from build123d import *

# Parameters (mm, degrees)
SKETCH_1_R          = 13.05
EXTRUDE_1_DEPTH     = 65.9
SKETCH_2_R          = 10.978194701
CUT_EXTRUDE_1_DEPTH = 0.5
SKETCH_3_R          = 5.021706909
EXTRUDE_2_DEPTH     = 0.5
CUT_EXTRUDE_START   = -0.2
SKETCH_4_R          = 8.048308781
SKETCH_4_R_2        = 5.021706909
CUT_EXTRUDE_2_DEPTH = 0.2


with BuildPart() as part:
    # 草图1 → 凸台-拉伸1 (new body)
    with BuildSketch(Plane(origin=(0, 0, 0), x_dir=(1, 0, 0), z_dir=(0, 1, 0))):
        with Locations(Location((0, 0, 0), (0, 0, 270))):
            Circle(SKETCH_1_R)
    extrude(amount=EXTRUDE_1_DEPTH)

    # 草图2 → 切除-拉伸1 (cut)
    with BuildSketch(Plane.XZ):
        with Locations(Location((0, 0, 0), (0, 0, 270))):
            Circle(SKETCH_2_R)
    extrude(amount=-CUT_EXTRUDE_1_DEPTH, mode=Mode.SUBTRACT)

    # 草图3 → 凸台-拉伸2 (add)
    with BuildSketch(Plane(origin=(0, 65.9, 0), x_dir=(1, 0, 0), z_dir=(0, 1, 0))):
        with Locations(Location((0, 0, 0), (0, 0, 270))):
            Circle(SKETCH_3_R)
    extrude(amount=EXTRUDE_2_DEPTH)

    # 草图4 → 切除-拉伸2 (cut)
    with BuildSketch(Plane(origin=(0, 65.9, 0), x_dir=(1, 0, 0), z_dir=(0, 1, 0)).offset(CUT_EXTRUDE_START)):
        with Locations(Location((0, 0, 0), (0, 0, 270))):
            Circle(SKETCH_4_R)
        with Locations(Location((0, 0, 0), (0, 0, 270))):
            Circle(SKETCH_4_R_2, mode=Mode.SUBTRACT)
    extrude(amount=CUT_EXTRUDE_2_DEPTH, mode=Mode.SUBTRACT)


solid = part.part
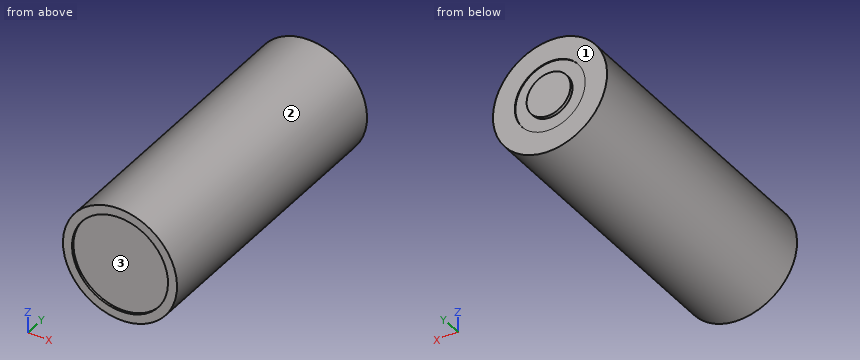
CAD build for the part. Positions are in the model's coordinates, mm. Face numbers are marked on the shaded views. Coordinates: 2 decimals unless noted, no trailing zeros. Order: outer loops, then holes, each group sorted by start corner. A loop starts at its lowest first (then second) coordinate and runs counter-clockwise, first axis right, second up.
Item 1: Band-saw the part on B-B on z = 4. List the corners of the cut face in (x, y).
Check sheet entries:
outline: (-12.42, 0) - (-10.22, 0) - (-10.22, 0.5) - (10.22, 0.5) - (10.22, 0) - (12.42, 0) - (12.42, 65.9) - (6.98, 65.9) - (6.98, 65.7) - (3.04, 65.7) - (3.04, 66.4) - (-3.04, 66.4) - (-3.04, 65.7) - (-6.98, 65.7) - (-6.98, 65.9) - (-12.42, 65.9) - close
Item 2: Band-saw the part on A-A on x = 1.75. List the corners of the cut face in (y, z).
Check sheet entries:
outline: (0, -12.93) - (65.9, -12.93) - (65.9, -7.86) - (65.7, -7.86) - (65.7, -4.71) - (66.4, -4.71) - (66.4, 4.71) - (65.7, 4.71) - (65.7, 7.86) - (65.9, 7.86) - (65.9, 12.93) - (0, 12.93) - (0, 10.84) - (0.5, 10.84) - (0.5, -10.84) - (0, -10.84) - close
Item 3: Drill centre lines: L1, parallel to X at y = 65.85, z = 0; L2, parallel to X at y = 0.3, z = 0; L3, parallel to Y at x = 6.25, z = 8. Where is each one in solid material? Low to high.
Check sheet entries:
L1: x = -13.05 to -8.05, -5.02 to 5.02, 8.05 to 13.05
L2: x = -13.05 to -10.98, 10.98 to 13.05
L3: y = 0.5 to 65.9
Item 4: Pin check, flat tips, straight feed: pin 1 Ø12 at (y, z) = (11, 4) entering from -X; pin 2 Ø3 at (x, z) = (-0.5, 4.5) entering from -Y; pin 3 Ø10 at (y, z) = (37, -10.5) entering from -X; pin 4 Ø8 at (x, z) = (8.5, 6) entering from +Y. Stop position of each tip, or through.
Check sheet entries:
pin 1: stops at x = -13.05
pin 2: stops at y = 0.5
pin 3: stops at x = -11.83
pin 4: stops at y = 65.9
Item 5: Two-plate mould, pull along X, no slides. Class the marked faces 1, 2 and 3: +X half, -X half, draft (parallel to the pull), parting line (faces both ways), or undercut.
Check sheet entries:
face 1: draft
face 2: parting line
face 3: undercut
Item 6: Band-saw the part on C-C on y = 41.5. List the corners of the cut face in (x, z), plus the area to 3 significant figures.
Check sheet entries:
outline: circle Ø26.1 at (0, 0)
area: 535 mm2
Item 7: Band-saw the part on D-D on z = -10.25. List the corners of the cut face in (x, y).
Check sheet entries:
outline: (-8.08, 0) - (-3.93, 0) - (-3.93, 0.5) - (3.93, 0.5) - (3.93, 0) - (8.08, 0) - (8.08, 65.9) - (-8.08, 65.9) - close
